Source: CAD feature listing. Evaluate the final solid. Frame: model axes, mm. A direction names the side the tool comes from. Give positions to 0.01 mm unless a question says otherwise; leave off trailing zeros. Write each loop counter-clockwise with the first axis right and the second up, starting at its lowest first coordinate (ties: lowest second). Pieces come first, ordered by that corner, then holes. Notation, with made-up numbers: (-38.5, -30.5) -> (-3.5, -30.5) arc R27 ccw to (-3.5, 6.5) -> close; hole circle Ø4 at (-15, 31.5). An arc over 180 degrees is marked (long way). Use a Markdown table: item, result. Add a question column.
```python
from build123d import *

# Parameters (mm, degrees)
SKETCH_1_W          = 28.5
SKETCH_1_H          = 21.5
EXTRUDE_1_DEPTH     = 13.2
FILLET_1_R          = 1
SKETCH_3_W          = 14
SKETCH_3_H          = 14
CUT_EXTRUDE_2_DEPTH = 2
SKETCH_4_W          = 15.8
SKETCH_4_H          = 15.8
CUT_EXTRUDE_3_DEPTH = 0.8
FILLET_2_R          = 1


with BuildPart() as part:
    # 草图1 → 凸台-拉伸1 (new body)
    with BuildSketch(Plane(origin=(0, 0, 0), x_dir=(1, 0, 0), z_dir=(0, 1, 0))):
        Rectangle(SKETCH_1_W, SKETCH_1_H)
    extrude(amount=EXTRUDE_1_DEPTH)

    # 圆角1
    fillet_1_edges = [part.edges().sort_by_distance(p)[0] for p in [
        (14.25, 6.6, 10.75),
        (-14.25, 6.6, 10.75),
        (-14.25, 6.6, -10.75),
        (14.25, 6.6, -10.75),
    ]]
    fillet(fillet_1_edges, radius=FILLET_1_R)

    # 草图3 → 切除-拉伸2 (cut)
    with BuildSketch(Plane(origin=(0, 13.2, 0), x_dir=(1, 0, 0), z_dir=(0, 1, 0))):
        Rectangle(SKETCH_3_W, SKETCH_3_H)
    extrude(amount=-CUT_EXTRUDE_2_DEPTH, mode=Mode.SUBTRACT)

    # 草图4 → 切除-拉伸3 (cut)
    with BuildSketch(Plane(origin=(0, 13.2, 0), x_dir=(1, 0, 0), z_dir=(0, 1, 0))):
        Rectangle(SKETCH_4_W, SKETCH_4_H)
    extrude(amount=-CUT_EXTRUDE_3_DEPTH, mode=Mode.SUBTRACT)

    # 圆角2
    fillet_2_edges = [part.edges().sort_by_distance(p)[0] for p in [
        (14.25, 0, 0),
        (0, 0, 10.75),
        (-14.25, 0, 0),
        (0, 0, -10.75),
        (13.957106781, 0, -10.457106781),
        (-13.957106781, 0, -10.457106781),
        (-13.957106781, 0, 10.457106781),
        (13.957106781, 0, 10.457106781),
    ]]
    fillet(fillet_2_edges, radius=FILLET_2_R)


solid = part.part
```
(1) Access query for faces 1 (the flat face through (-14.25, 7, 0)), 2 (the flat face through (-7.9, 13, 0)). Directions: +Z, -Z, +X, -X, +Y, -Y. A direction counts if a zero-diameter tool reaches every point of the face in a straight line with its end or side. Return the directions, or none.
(2) Cut plane C-C on z = 2. Return the cut outline in (x, y).
(3) Mould query, pull axis X, two halves, no side actions, for faces 3 (the cylindrical face through (0.185, 0.285, 10.449)), 4 (the flat face through (14.25, 7, 0)), 5 (the flat face through (0, 11.2, 0)). Classes: +X half, -X half, draft (parallel to the pull), parting line (faces both ways), or undercut.
(4) First-contact query: pin 1 Ø4.5 at (x, z) = (-3.5, 1.5) entering from +Y. Flat tip, straight axial feed; report the tip coordinate or a pass-through.
(5) Material intervals for L1, parallel to Z at x = 5.5, y = 11.5; L2, parallel to Y at x = 4.25, z = -0.5; L3, parallel to Y at x = -7.5, z = 4, sorted ascending.
(6) Cut plane B-B on x = 6. Return the cut outline in (y, z).
(7) Cut plane A-A on y = 12. Return the cut outline in (x, z).
Output:
| question | item | result |
|---|---|---|
| 1 | face 1 | +Z, -Z, -X, +Y, -Y |
| 1 | face 2 | +Y |
| 2 | outline | (-14.25, 1) arc R1 ccw to (-13.25, 0) -> (13.25, 0) arc R1 ccw to (14.25, 1) -> (14.25, 13.2) -> (7.9, 13.2) -> (7.9, 12.4) -> (7, 12.4) -> (7, 11.2) -> (-7, 11.2) -> (-7, 12.4) -> (-7.9, 12.4) -> (-7.9, 13.2) -> (-14.25, 13.2) -> close |
| 3 | face 3 | draft |
| 3 | face 4 | +X half |
| 3 | face 5 | undercut |
| 4 | pin 1 | y = 11.2 |
| 5 | L1 | -10.75 to -7, 7 to 10.75 |
| 5 | L2 | 0 to 11.2 |
| 5 | L3 | 0 to 12.4 |
| 6 | outline | (0, -9.75) arc R1 ccw to (1, -10.75) -> (13.2, -10.75) -> (13.2, -7.9) -> (12.4, -7.9) -> (12.4, -7) -> (11.2, -7) -> (11.2, 7) -> (12.4, 7) -> (12.4, 7.9) -> (13.2, 7.9) -> (13.2, 10.75) -> (1, 10.75) arc R1 ccw to (0, 9.75) -> close |
| 7 | outline | (-14.25, -9.75) arc R1 ccw to (-13.25, -10.75) -> (13.25, -10.75) arc R1 ccw to (14.25, -9.75) -> (14.25, 9.75) arc R1 ccw to (13.25, 10.75) -> (-13.25, 10.75) arc R1 ccw to (-14.25, 9.75) -> close; hole (-7, -7) -> (7, -7) -> (7, 7) -> (-7, 7) -> close |
